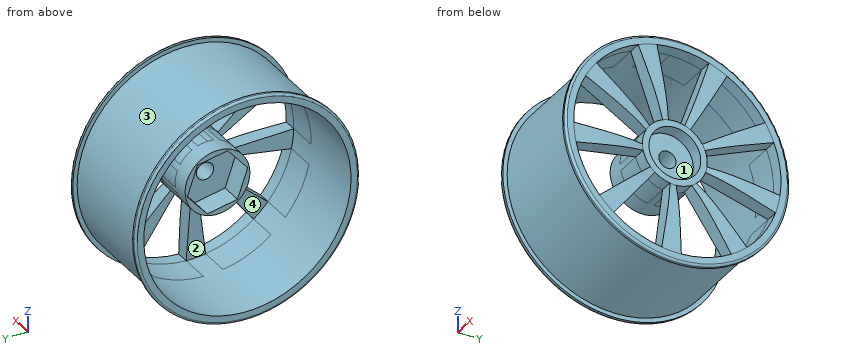
```python
from build123d import *
from build123d.topology import SkipClean

# Parameters (mm, degrees)
CUT_EXTRUDE2_DEPTH  = 10
CIRPATTERN1_COUNT   = 9
CUT_EXTRUDE9_DEPTH  = 5
BOSS_EXTRUDE2_START = -5
SKETCH7_R           = 6
BOSS_EXTRUDE2_DEPTH = 5
SKETCH8_R           = 2
CUT_EXTRUDE10_DEPTH = 6


with BuildPart() as part:
    # Sketch1 → Revolve1 (revolve)
    with BuildSketch(Plane(origin=(0, 0, 0), x_dir=(1, 0, 0), z_dir=(0, 1, 0)), mode=Mode.PRIVATE) as revolve1_sk:
        with BuildLine():
            Line((-13, 24), (10, 24))
            Line((10, 24), (9, 7.5))
            Line((9, 7.5), (-1, 7.5))
            Line((-1, 7.5), (-1, 6))
            Line((-1, 6), (12, 6))
            Line((12, 6), (12, 7.5))
            add(Edge.make_bspline(
                [(13, 24), (12.945427236, 18.482405329), (13.269747448, 12.974355238), (12, 7.5)],
                knots=[0, 0, 0, 0, 1, 1, 1, 1], degree=3))
            Line((13, 24), (13, 25.5))
            ThreePointArc((13, 25.5), (12.853553391, 25.853553391), (12.5, 26))
            Line((12.5, 26), (12, 26))
            Line((12, 26), (12, 25))
            Line((12, 25), (-12, 25))
            Line((-12, 25), (-12, 26))
            Line((-12, 26), (-12.5, 26))
            ThreePointArc((-12.5, 26), (-12.853553391, 25.853553391), (-13, 25.5))
            Line((-13, 25.5), (-13, 24))
        make_face()
    revolve(revolve1_sk.sketch.rotate(Axis((-89.555555556, 0, 0), (1, 0, 0)), 180), axis=Axis((-89.555555556, 0, 0), (1, 0, 0)))

    # Sketch2 → Cut-Extrude2 (cut)
    with BuildSketch(Plane(origin=(13, 0, 0), x_dir=(0, 0, -1), z_dir=(1, 0, 0))):
        with BuildLine():
            Line((-2.731619252, 6.984859072), (-8.741181606, 22.351549032))
            ThreePointArc((-8.741181606, 22.351549032), (-2.83241408, 23.832277073), (3.258818394, 23.777722824))
            Line((3.258818394, 23.777722824), (1.018380748, 7.430538382))
            ThreePointArc((1.018380748, 7.430538382), (-0.8851294, 7.447586585), (-2.731619252, 6.984859072))
        make_face()
    cut_extrude2 = extrude(amount=-CUT_EXTRUDE2_DEPTH, mode=Mode.SUBTRACT)

    # CirPattern1: Cut-Extrude2 ×9 about axis
    with SkipClean():  # the faces are left unmerged after this step: merging them gives an invalid solid
        cirpattern1_axis = Axis((0, 0, 0), (1, 0, 0))
        for i in range(1, CIRPATTERN1_COUNT):
            add(cut_extrude2.rotate(cirpattern1_axis, i * 360 / CIRPATTERN1_COUNT), mode=Mode.SUBTRACT)
    add(part.part.scale(1), mode=Mode.REPLACE)  # the faces are merged on a copy

    # Sketch6 → Cut-Extrude9 (cut)
    with BuildSketch(Plane.ZY.offset(1)):
        Polygon((-5.409909398, -4.629762059), (1.304536857, -7), (6.714446255, -2.370237941), (5.409909398, 4.629762059), (-1.304536857, 7), (-6.714446255, 2.370237941), align=None)
    extrude(amount=-CUT_EXTRUDE9_DEPTH, mode=Mode.SUBTRACT)

    # Sketch7 → Boss-Extrude2 (add)
    with BuildSketch(Plane.ZY.offset(-4).offset(BOSS_EXTRUDE2_START)):
        Circle(SKETCH7_R)
    extrude(amount=BOSS_EXTRUDE2_DEPTH)

    # Sketch8 → Cut-Extrude10 (cut)
    with SkipClean():  # the faces are left unmerged after this step: merging them gives an invalid solid
        with BuildSketch(Plane(origin=(9, 0, 0), x_dir=(0, 0, -1), z_dir=(1, 0, 0))):
            Circle(SKETCH8_R)
        extrude(amount=-CUT_EXTRUDE10_DEPTH, mode=Mode.SUBTRACT)


solid = part.part
```
CAD build for the part. Positions are in the model's coordinates, mm. Face numbers are marked on the shaded views. A direction names the side the tool comes from. Coordinates: 2 decimals unless noted, no trailing zeros. Order: outer loops, then holes, each group sorted by start corner. A loop starts at its lowest first (then second) coordinate and runs counter-clockwise, first axis right, second up. Notation, with made-up numbers: (77.5, 23) -> (97.5, 23) arc R32 ccw to (97.5, 57) -> close; hole circle Ø11 at (53, 83.5). An arc over 180 degrees is marked (long way). Use one line per item in the form item = value. Start each with the question number.
1) Drill centre lines: L1, parallel to Y at x = 10.55, z = 0; L2, parallel to Y at x = 6.05, z = 0; L3, parallel to Z at x = 10.5, y = 19.5. Where is each one in solid material? Low to high. Write a range as [from, to].
2) Tool access for the marked faces 1 and 2: list every direction of +Z, -Z, +X, -X, +Y, -Y with a clear straight run to the whole face (end or side of a thin tool).
3) Drop flat-ended pins along their axis: pin 1 (5 mm diameter, centred on y = 10.5, z = 7.5, fed in from +X); pin 2 (3 mm diameter, centred on x = 1, y = -19, fed in from -Z); pin 3 (15.5 mm diameter, centred on y = 0, z = 0, fed in from -X). Give the stop position or say it passes through.
4) Pull direction Z, two halves, no side cores. Call the marked faces 3 and 4: +Z half, -Z half, draft (parallel to the pull), parting line (faces both ways), or undercut.
5) Band-saw the part on C-C on z = 20. State how many separate pieces and enclosed holes the cut face has, then the cut area to 3 significant figures.
6) Band-saw the part on A-A on x = 1.5. Give the cut face in (y, z), then the cut area to 3 significant figures.
7) Band-saw the part on B-B on x = 7.5. Give the cut face in (y, z), then the cut area to 3 significant figures.
Entries:
q1.L1 = [-25, -24], [-7.5, -6], [6, 7.5], [24, 25]
q1.L2 = [-25, -24], [-7.5, -2], [2, 7.5], [24, 25]
q1.L3 = [-15.64, -13.99], [-6.58, -2.67], [7.63, 12.28], [13.99, 15.64]
q2.face_1 = +X
q2.face_2 = -X
q3.pin_1 = 12.94
q3.pin_2 = -17.85
q3.pin_3 = -1
q4.face_3 = parting line
q4.face_4 = undercut
q5.separate_pieces = 4
q5.enclosed_holes = 0
q5.area = 124 mm2
q6.outline = circle Ø50 at (0, 0); circle Ø15 at (0, 0); hole circle Ø48 at (0, 0); hole (-7, 1.3) -> (-4.63, -5.41) -> (2.37, -6.71) -> (7, -1.3) -> (4.63, 5.41) -> (-2.37, 6.71) -> close
q6.area = 199 mm2
q7.outline = circle Ø50 at (0, 0); circle Ø15 at (0, 0); hole circle Ø48 at (0, 0); hole circle Ø4 at (0, 0)
q7.area = 318 mm2
